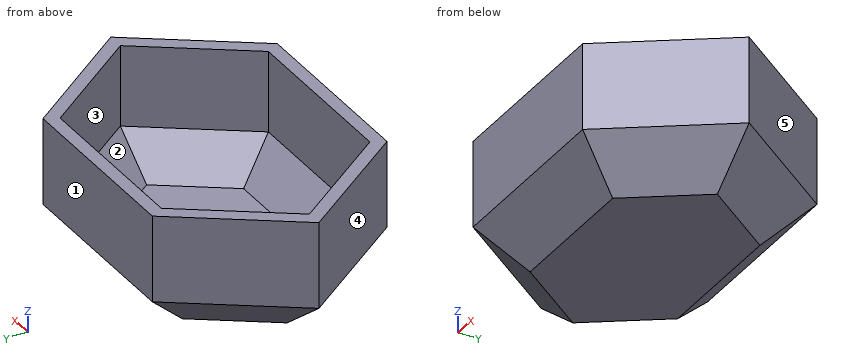
```python
from build123d import *

# Parameters (mm, degrees)
F1_DEPTH = 76.2
F2_SIZE  = 25.4
F3_T     = -7.62


with BuildPart() as f1:
    # F0 (on Top) → F1 (new body)
    with BuildSketch(Plane.XY):
        Polygon((-52.830831, 42.997032), (0, 42.997032), (53.74952, 42.997032), (53.74952, 68.397032), (-52.830831, 68.397032), align=None)
        Polygon((-75.556472, 0), (-52.830831, 42.997032), (-52.830831, 68.397032), (-100.956472, 0), align=None)
        Polygon((53.74952, 68.397032), (53.74952, 42.997032), (76.477893, 0), (101.877893, 0), align=None)
        Polygon((53.74952, 42.997032), (0, 42.997032), (-52.830831, 42.997032), (-75.556472, 0), (-52.830831, -43.0022), (53.74952, -43.0022), (76.477893, 0), align=None)
        Polygon((101.877893, 0), (76.477893, 0), (53.74952, -43.0022), (53.74952, -68.4022), align=None)
        Polygon((53.74952, -43.0022), (-52.830831, -43.0022), (-53.135242, -68.4022), (53.74952, -68.4022), align=None)
        Polygon((-52.830831, -43.0022), (-75.556472, 0), (-100.956472, 0), (-53.135242, -68.4022), align=None)
    extrude(amount=F1_DEPTH)

    # F2
    f2_edges = [f1.edges().sort_by_distance(p)[0] for p in [
        (0.459345, 68.397032, 0),
        (-76.893652, 34.198516, 0),
        (-77.045857, -34.2011, 0),
        (0.307139, -68.4022, 0),
        (77.813707, -34.2011, 0),
        (77.813707, 34.198516, 0),
    ]]
    chamfer(f2_edges, length=F2_SIZE)

    # F3
    f3_openings = [f1.faces().sort_by_distance(p)[0] for p in [
        (0.425958, -0.024737, 76.2),
    ]]
    offset(amount=F3_T, openings=f3_openings)


solid = f1.part
```
The listing builds one solid part. Answer for the finished solid, in the listing's coordinates (mm). Face numbers are marked on the shaded views. A direction names the side the tool comes from. Coordinates: 2 decimals unless noted, no trailing zeros. Write each loop counter-clockwise with the first axis right and the second up, starting at its lowest first coordinate (ties: lowest second). Pieces come first, ordered by that corner, then holes.
Q1. Section A-A, the plane z = 37.5 is taken. Write down the section's boundary in (x, y), then the cut area to 3 significant figures.
Returned:
outline: (-100.96, 0) - (-53.14, -68.4) - (53.75, -68.4) - (101.88, 0) - (53.75, 68.4) - (-52.83, 68.4) - close; hole (-91.65, -0.01) - (-49.16, -60.78) - (49.79, -60.78) - (92.56, 0) - (49.79, 60.78) - (-48.88, 60.78) - close
area: 3,970 mm2
Q2. Given P1, Ø5, axis at x = 73.5, z = 38, coming from the +Y side; P2, Ø10, axis at y = 8, z = 67, coming from the -X side; P3, Ø6, axis at x = -78, y = -10.5, coming from the +Z side, each flat-ended and moving along its own axis, determine where each tip first touches the part or whether it passes through.
Returned:
P1: stops at y = 43.88
P2: stops at x = -98.85
P3: stops at z = 26.38
Q3. Which of the six approach directions +Z, -Z, +X, -X, +Y, -Y give full straight-line access (tool end or side, diameter ignored) to the marked faces 1 and 2?
Returned:
face 1: +Z, -Z, +X, -X, +Y
face 2: +Z
Q4. Section C-C, the plane y = 37 is taken. Write down the section's boundary in (x, z).
Returned:
outline: (-74.92, 25.4) - (-43.86, 0) - (44.78, 0) - (75.84, 25.4) - (75.84, 76.2) - (66.52, 76.2) - (66.52, 28.56) - (40.92, 7.62) - (-40.01, 7.62) - (-65.61, 28.56) - (-65.61, 76.2) - (-74.92, 76.2) - close
Q5. Section D-D, the plane x = -73.5 is taken. Write down the section's boundary in (y, z), then the cut area to 3 significant figures.
Returned:
outline: (-39.27, 25.4) - (-0.04, 2.92) - (39.02, 25.4) - (39.02, 76.2) - (25.78, 76.2) - (25.78, 28.56) - (-0.04, 13.7) - (-25.97, 28.56) - (-25.97, 76.2) - (-39.27, 76.2) - close
area: 2,010 mm2
Q6. Find the intervals of material crossed by line 1 along Y through (x, z) = (47, 46); line 2 along Y through (x, z) = (-42, 13); line 3 along X through (y, z) = (-18.5, 42), in increasing order.
Returned:
line 1: y = -68.4 to -60.78, 60.78 to 68.4
line 2: y = -56 to -43.88, 43.51 to 56
line 3: x = -88.02 to -78.73, 79.54 to 88.86
Q7. Section B-B, the plane x = 26 is taken. Write down the section's boundary in (y, z).
Returned:
outline: (-68.4, 25.4) - (-43, 0) - (43, 0) - (68.4, 25.4) - (68.4, 76.2) - (60.78, 76.2) - (60.78, 28.56) - (39.84, 7.62) - (-39.85, 7.62) - (-60.78, 28.56) - (-60.78, 76.2) - (-68.4, 76.2) - close
Q8. The mould has two halves that part along Y. Classify the marked faces 3, 4 and 5: released by +Y, released by -Y, zero draft, split by the parting line, or undercut.
Returned:
face 3: undercut
face 4: released by -Y
face 5: released by +Y
